Could you check a few things on this drawing? It's one solid part, dimensions in mm from its lowest x, y, z. Round coordinates to 2 decimals unless told otherwise and drop trailing zeros. Write each loop counter-clockwise with the first axis right and the second up, starting at its lowest first coordinate (ties: lowest second). Pieces come first, ordered by that corner, then holes. Notation, with made-up numbers: (-11, 89.5) -> (-4, 89.5) arc R10 ccw to (-4, 100.5) -> close; hole circle Ø10 at (-32.75, 19.25). An arc over 180 degrees is marked (long way). Return JSON: item names as keys, results as strings.
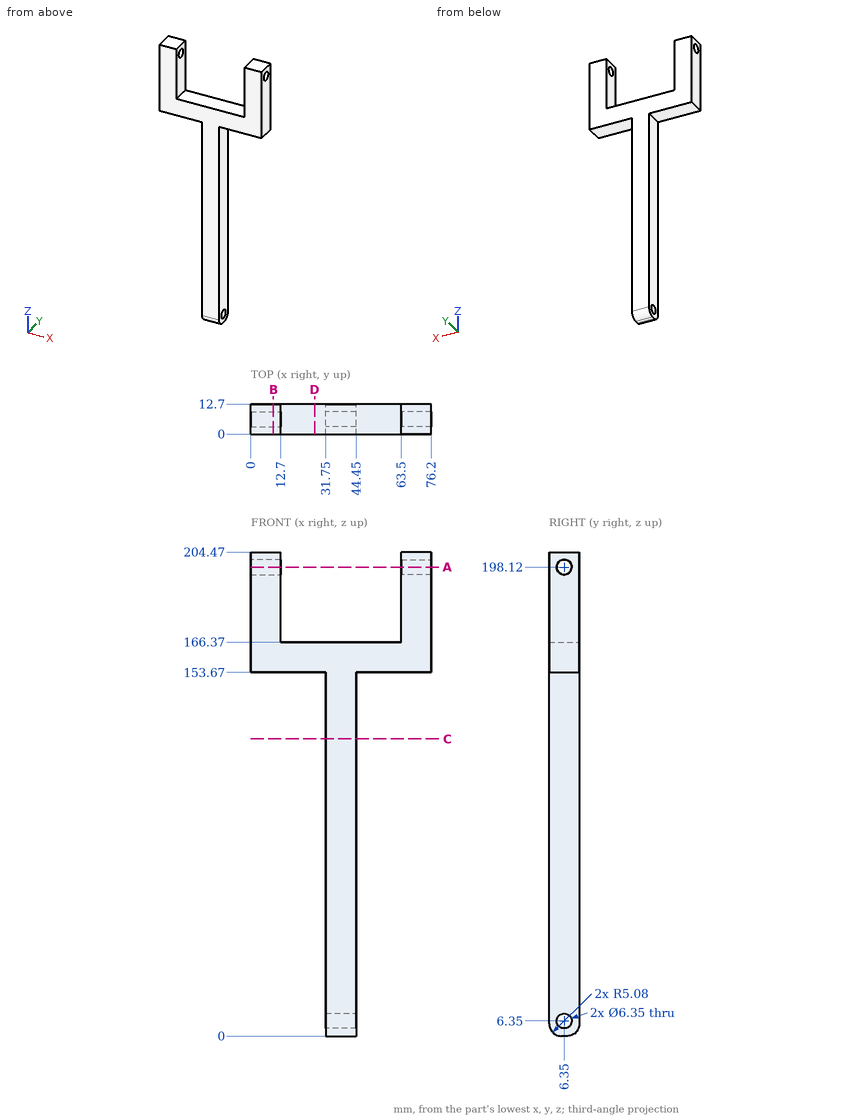
1) Will these pins go through, and if not, where does the flat tip stop? pin 1 Ø4 at (x, y) = (18.5, 4) entering from -Z; pin 2 Ø1.5 at (y, z) = (2.5, 62) entering from +X; pin 3 Ø1 at (x, y) = (43, 2.5) entering from +Z.
Return value:
{"pin 1": "z = 153.67", "pin 2": "x = 44.45", "pin 3": "z = 166.37"}
2) I want a section at A-A, the plane z = 198.12. Please give me the cut outline in (x, y) (3 decimals), and give its area (3 significant figures).
Return value:
{"outline": "(0, 0) -> (12.7, 0) -> (12.7, 3.175) -> (0, 3.175) -> close; (0, 9.525) -> (12.7, 9.525) -> (12.7, 12.7) -> (0, 12.7) -> close; (63.5, 0) -> (76.2, 0) -> (76.2, 3.175) -> (63.5, 3.175) -> close; (63.5, 9.525) -> (76.2, 9.525) -> (76.2, 12.7) -> (63.5, 12.7) -> close", "area": "161 mm²"}
3) If I drill on probe 1 along X at (y, z) = (8.5, 191); probe 2 along Y at (x, z) = (8, 198.12) (3 decimals); probe 3 along Z at (x, y) = (38.5, 6.5), over which ranges is the centre line in solid material (lowest first)? Write a range as [from, to].
Return value:
{"probe 1": "[0, 12.7], [63.5, 76.2]", "probe 2": "[0, 3.175], [9.525, 12.7]", "probe 3": "[0, 3.18], [9.52, 166.37]"}
4) I want a section at C-C, the plane z = 125.5. Please give me the cut outline in (x, y), and give its area (3 significant figures).
Return value:
{"outline": "(31.75, 0) -> (44.45, 0) -> (44.45, 12.7) -> (31.75, 12.7) -> close", "area": "161 mm²"}
5) I want a section at D-D, the plane x = 27. Please give me the cut outline in (y, z), and give its area (3 significant figures).
Return value:
{"outline": "(0, 153.67) -> (12.7, 153.67) -> (12.7, 166.37) -> (0, 166.37) -> close", "area": "161 mm²"}
6) I want a section at B-B, the plane x = 9.5. Please give me the cut outline in (y, z) (3 decimals), and give its area (3 significant figures).
Return value:
{"outline": "(0, 153.67) -> (12.7, 153.67) -> (12.7, 204.47) -> (0, 204.47) -> close; hole circle Ø6.35 at (6.35, 198.12)", "area": "613 mm²"}
